Autodesk Inventor part; units mm, degrees
ref_plane "YZ Plane" through (0, 0, 0) normal (1, 0, 0) x (0, 1, 0)
ref_plane "XZ Plane" through (0, 0, 0) normal (0, 1, 0) x (-1, 0, 0)
ref_plane "XY Plane" through (0, 0, 0) normal (0, 0, 1) x (1, 0, 0)
sketch "Sketch1" plane through (0, 0, 0) normal (0, 0, 1) x (1, 0, 0)
  circle A0 centre (0, 0) radius 50
  line L0 (-16.25, -47.2857) -> (16.25, -47.2857)
  dimension "d1" = 32.5
  dimension "d2" = 100
extrude "Extrusion1" add sketch "Sketch1" along normal blind 0.525 contours A0 L0 picked at (-0.3738, -14.8613)
sketch "Sketch2" plane through (0, 0, 0.525) normal (0, 0, 1) x (1, 0, 0)
  arc A0 (16.25, -47.2857) -> (-16.25, -47.2857) centre (0, 0) ccw
  line L0 (-0.35, 0.35) -> (-0.3, 0.35)
  line L1 (-0.3, 0.35) -> (-0.3, 0.3)
  line L2 (-0.3, 0.3) -> (-0.25, 0.3)
  line L3 (-0.25, 0.3) -> (-0.25, 0.25)
  line L4 (-0.25, 0.25) -> (-0.3, 0.25)
  line L5 (-0.3, 0.25) -> (-0.3, 0.2)
  line L6 (-0.3, 0.2) -> (-0.35, 0.2)
  line L7 (-0.35, 0.2) -> (-0.35, 0.25)
  line L8 (-0.35, 0.25) -> (-0.4, 0.25)
  line L9 (-0.4, 0.25) -> (-0.4, 0.3)
  line L10 (-0.4, 0.3) -> (-0.35, 0.3)
  line L11 (-0.35, 0.3) -> (-0.35, 0.35)
  dimension "d5" = 0.05
  dimension "d6" = 0.25
  dimension "d7" = 0.25
extrude "Extrusion2" cut sketch "Sketch2" against normal blind 0.025
chamfer "Chamfer2" distance 0.0249 angle 35.3 12 edges at (-0.325, 0.35, 0.5) (-0.35, 0.325, 0.5) (-0.375, 0.3, 0.5) (-0.4, 0.275, 0.5) (-0.375, 0.25, 0.5) (-0.35, 0.225, 0.5) (-0.325, 0.2, 0.5) (-0.3, 0.225, 0.5) (-0.275, 0.25, 0.5) (-0.25, 0.275, 0.5) (-0.275, 0.3, 0.5) (-0.3, 0.325, 0.5) measured on face at (-0.3833, 0.2833, 0.5)
properties part number "combdrive-test" material "Silicon"
Design review of the part built by this model. Coordinates are the model's own, in mm. Coordinates: 2 decimals unless noted, no trailing zeros. Order: outer loops, then holes, each group sorted by start corner. A loop starts at its lowest first (then second) coordinate and runs counter-clockwise, first axis right, second up. Notation, with made-up numbers: M 29,-6.5 L 88,-6.5 A20 ccw 88,29.5 Z; hole C -39,-22.75 d1. An arc over 180 degrees is marked long. Answer as a JSON object with one key per item and string values. Group by question number.
1) Add section A-A, the plane z = 0.2. Write out the cut boundary in (x, y), then the cut area to 3 significant figures.
2) Add section B-B, the plane y = 44.5. Write out the cut boundary in (x, z) (3 decimals).
3) Add section C-C, the plane x = -27.5. Write out the cut boundary in (y, z) (3 decimals), then the cut area to 3 significant figures.
4) Wall thickness on L1, parallel to Y at x = 0.5, z = 0.2; L2, parallel to X at y = -39.5, z = 0.4; L3, parallel to X at y = -10.5, z = 0.15: over which ranges is each line inside the solid? List them lowest first.
Computed values:
{
 "1": {"outline": "M -16.25,-47.29 L 16.25,-47.29 A50 ccw long Z", "area": "7,790 mm^2"},
 "2": {"outline": "M -22.798,0 L 22.798,0 L 22.798,0.525 L -22.798,0.525 Z"},
 "3": {"outline": "M -41.758,0 L 41.758,0 L 41.758,0.525 L -41.758,0.525 Z", "area": "43.8 mm^2"},
 "4": {"L1": "y = -47.29 to 50", "L2": "x = -30.66 to 30.66", "L3": "x = -48.89 to 48.89"}
}
